Source: CAD feature listing. Evaluate the final solid. Frame: model axes, mm. Face numbers are marked on the shaded views. A direction names the side the tool comes from. Round coordinates to 2 decimals unless told otherwise and drop trailing zeros. Write each loop counter-clockwise with the first axis right and the second up, starting at its lowest first coordinate (ties: lowest second). Pieces come first, ordered by that corner, then holes. Notation, with made-up numbers: M 35,-37 L 69,-37 A30 cw 69,-3 Z; hole C 24.25,18.5 d3. An arc over 180 degrees is marked long. Put each result on its own line as item: value. Start each with the question number.
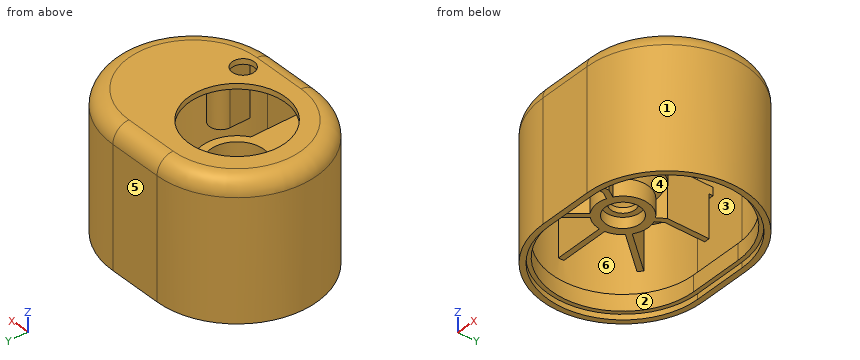
```python
from build123d import *

# Parameters (mm, degrees)
EXTRUDE_1_DEPTH     = 51
FILLET_1_R          = 6
SHELL_1_T           = -2
SKETCH_3_R          = 18
CUT_EXTRUDE_1_DEPTH = 72.421285343
SKETCH_5_R          = 4.1
CUT_EXTRUDE_2_DEPTH = 4
EXTRUDE_START       = -2
EXTRUDE_2_DEPTH     = 6
EXTRUDE_START_2     = -3
EXTRUDE_3_DEPTH     = 3
EXTRUDE_32_REACH    = 62.465
EXTRUDE_36_REACH    = 62.465
EXTRUDE_37_REACH    = 62.465
SKETCH_14_W         = 19.811684382
SKETCH_14_H         = 2
EXTRUDE_4_DEPTH     = 24.8
HOLE_WIZARD_1_D     = 2
HOLE_WIZARD_1_DEPTH = 20


# Read off the part's stored shape, not the designer's step: the extrude step
with BuildPart() as part:
    # Sketch 2 → Extrude 1 (new body)
    with BuildSketch(Plane.XY):
        with BuildLine():
            Line((-10, 30), (10, 30))
            ThreePointArc((10, 30), (40, 0), (10, -30))
            Line((10, -30), (-10, -30))
            ThreePointArc((-10, -30), (-40, 0), (-10, 30))
        make_face()
    extrude(amount=EXTRUDE_1_DEPTH)

    # Fillet 1
    fillet_1_edges = [part.edges().sort_by_distance(p)[0] for p in [
        (40, 0, 51),
        (0, 30, 51),
        (-40, 0, 51),
        (0, -30, 51),
    ]]
    fillet(fillet_1_edges, radius=FILLET_1_R)

    # Shell 1
    shell_1_openings = [part.faces().sort_by_distance(p)[0] for p in [
        (0, 0, 0),
    ]]
    offset(amount=SHELL_1_T, openings=shell_1_openings, kind=Kind.INTERSECTION)

    # Sketch 3 → Cut-Extrude 1 (cut, through all)
    with BuildSketch(Plane.XY.offset(51)):
        with Locations((-10, 0)):
            Circle(SKETCH_3_R)
    extrude(amount=-CUT_EXTRUDE_1_DEPTH, mode=Mode.SUBTRACT)

    # Sketch 5 → Cut-Extrude 2 (cut)
    with BuildSketch(Plane.XY.offset(51)):
        with Locations((9, -18)):
            Circle(SKETCH_5_R)
    extrude(amount=-CUT_EXTRUDE_2_DEPTH, mode=Mode.SUBTRACT)

    # Sketch 6 → Extrude 2 (add)
    with BuildSketch(Plane(origin=(0, 0, 0), x_dir=(-1, 0, 0), z_dir=(0, 0, -1)).offset(EXTRUDE_START)):
        with BuildLine():
            Line((10, 28), (-10, 28))
            ThreePointArc((-10, 28), (-38, 0), (-10, -28))
            Line((-10, -28), (10, -28))
            ThreePointArc((10, -28), (38, 0), (10, 28))
        make_face()
        with BuildLine():
            Line((10, 26.5), (-10, 26.5))
            ThreePointArc((-10, 26.5), (-36.5, 0), (-10, -26.5))
            Line((-10, -26.5), (10, -26.5))
            ThreePointArc((10, -26.5), (36.5, 0), (10, 26.5))
        make_face(mode=Mode.SUBTRACT)
    extrude(amount=-EXTRUDE_2_DEPTH)



with BuildPart() as body_2:
    # Sketch 4 → Revolve 1 (revolve)
    with BuildSketch(Plane(origin=(0, 0, 0), x_dir=(1, 0, 0), z_dir=(0, 1, 0))):
        Polygon((-20, -36), (-20, -30), (-18, -30), (-18, -28), (-14.5, -23), (-14.5, -21), (-16.5, -21), (-16.5, -17), (-19.5, -17), (-19.5, -23.167682505), (-23, -28.167682505), (-23, -36), align=None)
    revolve(axis=Axis((-10, 0, 0), (0, 0, 1)))


with BuildPart() as part_1:
    add(part.part)

    add(body_2.part)  # Extrude 3 merges body 2
    # Sketch 7 → Extrude 3 (add)
    with BuildSketch(Plane.XY.offset(36).offset(EXTRUDE_START_2)):
        with BuildLine():
            Line((-3, 7.141428429), (-3, 28))
            Line((-3, 28), (-10, 28))
            ThreePointArc((-10, 28), (-38, 0), (-10, -28))
            Line((-10, -28), (-3, -28))
            Line((-3, -28), (-3, -7.141428429))
            ThreePointArc((-3, -7.141428429), (-20, 0), (-3, 7.141428429))
        make_face()
    extrude(amount=EXTRUDE_3_DEPTH)

    # Sketch 12 → Extrude 32 (add, up to next)
    with BuildSketch(Plane(origin=(0, 0, 17), x_dir=(-1, 0, 0), z_dir=(0, 0, -1)), mode=Mode.PRIVATE) as extrude_32_sk1:
        Polygon((3, -28), (3, -10.95445115), (6.5, -5.477225575), (8.185300177, -6.554148652), (5, -11.538893679), (5, -28), align=None)
    extrude_32_tool1 = extrude(extrude_32_sk1.sketch, amount=-EXTRUDE_32_REACH, mode=Mode.PRIVATE) - part_1.part
    add(extrude_32_tool1.solids().sort_by_distance((-4.44371, -16.649108, 17))[0])

    # Sketch 12_6 → Extrude 36 (add, up to next)
    with BuildSketch(Plane(origin=(0, 0, 17), x_dir=(-1, 0, 0), z_dir=(0, 0, -1)), mode=Mode.PRIVATE) as extrude_36_sk1:
        Polygon((3, 26.5), (3, 10.95445115), (6.5, 5.477225575), (8.185300177, 6.554148652), (5, 11.538893679), (5, 26.5), align=None)
    extrude_36_tool1 = extrude(extrude_36_sk1.sketch, amount=-EXTRUDE_36_REACH, mode=Mode.PRIVATE) - part_1.part
    add(extrude_36_tool1.solids().sort_by_distance((-4.474722, 15.908171, 17))[0])

    # Sketch 14 → Extrude 37 (add, up to next)
    with BuildSketch(Plane(origin=(0, 0, 17), x_dir=(-1, 0, 0), z_dir=(0, 0, -1)), mode=Mode.PRIVATE) as extrude_37_sk1:
        with Locations((28.094157809, 0)):
            Rectangle(SKETCH_14_W, SKETCH_14_H)
    extrude_37_tool1 = extrude(extrude_37_sk1.sketch, amount=-EXTRUDE_37_REACH, mode=Mode.PRIVATE) - part_1.part
    # Sketch 14 → Extrude 37 (add, up to next)
    with BuildSketch(Plane(origin=(0, 0, 17), x_dir=(-1, 0, 0), z_dir=(0, 0, -1)), mode=Mode.PRIVATE) as extrude_37_sk2:
        Polygon((16.029392267, 5.629826068), (28.764097514, 20.806456798), (27.232008628, 22.092032017), (14.49730338, 6.915401287), align=None)
    extrude_37_tool2 = extrude(extrude_37_sk2.sketch, amount=-EXTRUDE_37_REACH, mode=Mode.PRIVATE) - part_1.part
    # Sketch 14 → Extrude 37 (add, up to next)
    with BuildSketch(Plane(origin=(0, 0, 17), x_dir=(-1, 0, 0), z_dir=(0, 0, -1)), mode=Mode.PRIVATE) as extrude_37_sk3:
        Polygon((14.49730338, -6.915401287), (27.232008628, -22.092032017), (28.764097514, -20.806456798), (16.029392267, -5.629826068), align=None)
    extrude_37_tool3 = extrude(extrude_37_sk3.sketch, amount=-EXTRUDE_37_REACH, mode=Mode.PRIVATE) - part_1.part
    add(extrude_37_tool1.solids().sort_by_distance((-28.094158, 0, 17))[0])
    add(extrude_37_tool2.solids().sort_by_distance((-21.6307, 13.860929, 17))[0])
    add(extrude_37_tool3.solids().sort_by_distance((-21.6307, -13.860929, 17))[0])

    # Extrude 4 outline → Extrude 4 (add)
    with BuildSketch(Plane.XY.offset(24.2)):
        with BuildLine():
            ThreePointArc((16.890769815, -27.138852064), (21.143513187, -25.687002819), (25.109230185, -23.573526745))
            Line((25.109230185, -23.573526745), (25.109230185, -19.500000001))
            ThreePointArc((25.109230185, -19.500000001), (21.000000001, -15.390769815), (16.890769815, -19.5))
            Line((16.890769815, -19.5), (16.890769815, -27.138852064))
        make_face()
        with BuildLine():
            ThreePointArc((16.890769815, 19.5), (21.000000001, 15.390769815), (25.109230185, 19.500000001))
            Line((25.109230185, 19.500000001), (25.109230185, 23.573526745))
            ThreePointArc((25.109230185, 23.573526745), (21.143513187, 25.687002819), (16.890769815, 27.138852064))
            Line((16.890769815, 27.138852064), (16.890769815, 19.5))
        make_face()
    extrude(amount=EXTRUDE_4_DEPTH)

    # Hole Wizard 1
    with Locations(Plane(origin=(0, 0, 24.2), x_dir=(-1, 0, 0), z_dir=(0, 0, -1))):
        with Locations((-21, 19.5), (-21, -19.5)):
            Hole(HOLE_WIZARD_1_D / 2, depth=HOLE_WIZARD_1_DEPTH)


solid = part_1.part
```
(1) Pull-direction query (Z, two-part tool) for the marked faces 4, 5 and 6; classes: +Z half, -Z half, draft (parallel to the pull), parting line (faces both ways), or undercut.
(2) Section query C-C (y = 0). Count the separate pieces of the cut face and the enclosed holes in it, and give its area (3 significant figures).
(3) Access query for the marked faces 1, 2 and 3. Directions: +Z, -Z, +X, -X, +Y, -Y. A direction counts if a zero-diameter tool reaches every point of the face in a straight line with its end or side. Return the directions, or none.
(4) Section query A-A (z = 11). Return loops of the section in (x, y), and give its area (3 significant figures).
(5) Contact query for flat-ended pins moving along their axis: P1, Ø13.5, axis at y = 19.5, z = 28.5, coming from the +X side; P2, Ø5, axis at x = 15, z = 34.5, coming from the +Y side; P3, Ø1.5, axis at y = 8, z = 15, coming from the +X side; P4, Ø5, axis at x = 9, y = -18, coming from the -Z side. Output: stop coordinate, or through.
(6) Section query B-B (x = 9). Return loops of the section in (y, z).
(7) Ray query, line 1 along X through (y, z) = (0, 21.6); line 2 along X through (y, z) = (0, 29.6); line 3 along Y through (x, z) = (-10, 22.4). Return the intervals inside material, ascending.
Entries:
1. face 4: -Z half
1. face 5: draft
1. face 6: undercut
2. separate pieces: 3
2. enclosed holes: 0
2. area: 758 mm2
3. face 1: +Z, -Z, +X
3. face 2: -Z
3. face 3: none
4. outline: M -10,-30 L 10,-30 A30 ccw 10,30 L -10,30 A30 ccw Z; hole M -10,-28 L 10,-28 A28 ccw 10,28 L -10,28 A28 ccw Z
4. area: 444 mm2
5. P1: x = 37.16
5. P2: y = 29.9
5. P3: x = 39.11
5. P4: through
6. outline: M -30,0 L -28,0 L -28,2 L -26.5,2 L -26.5,8 L -28,8 L -28,45 A4 cw -24,49 L -22.1,49 L -22.1,51 L -24,51 A6 ccw -30,45 Z; M -13.9,49 L 24,49 A4 cw 28,45 L 28,8 L 26.5,8 L 26.5,2 L 28,2 L 28,0 L 30,0 L 30,45 A6 ccw 24,51 L -13.9,51 Z
7. line 1: -40 to -14.5, -5.5 to -0.5, 38 to 40
7. line 2: -40 to -18, -2 to 3, 38 to 40
7. line 3: -30 to -28, -9.5 to -4.5, 4.5 to 9.5, 28 to 30
